Part model, mm, in its own coordinate system. Face numbers are marked on the shaded views. A direction names the side the tool comes from. Round coordinates to 2 decimals unless told otherwise and drop trailing zeros. Write each loop counter-clockwise with the first axis right and the second up, starting at its lowest first coordinate (ties: lowest second). Pieces come first, ordered by that corner, then holes.
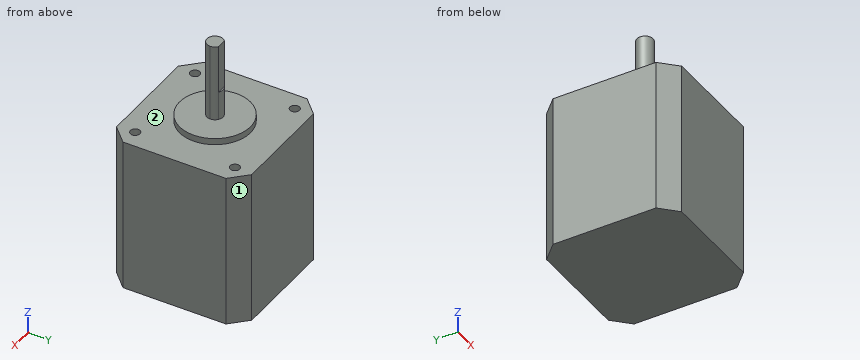
from build123d import *

# Parameters (mm, degrees)
SKETCH1_R           = 11
SKETCH1_R_2         = 1.5
SKETCH1_R_3         = 2.5
BOSS_EXTRUDE1_DEPTH = 48
SKETCH1_3_R         = 11
SKETCH1_3_R_2       = 2.5
BOSS_EXTRUDE2_DEPTH = 2
BOSS_EXTRUDE3_DEPTH = 26
BOSS_EXTRUDE4_DEPTH = 11
SKETCH1_6_R         = 1.5
CUT_EXTRUDE1_DEPTH  = 5


with BuildPart() as part:
    # Sketch1 → Boss-Extrude1 (new body)
    # profile 1 of 10: a face of its own
    with BuildSketch(Plane.XY):
        Polygon((-16, -21), (-21, -16), (-21, 16), (-16, 21), (16, 21), (21, 16), (21, -16), (16, -21), align=None)
        Circle(SKETCH1_R, mode=Mode.SUBTRACT)
        with Locations((15.5, -15.5)):
            Circle(SKETCH1_R_2, mode=Mode.SUBTRACT)
        with Locations((-15.5, -15.5)):
            Circle(SKETCH1_R_2, mode=Mode.SUBTRACT)
        with Locations((15.5, 15.5)):
            Circle(SKETCH1_R_2, mode=Mode.SUBTRACT)
        with Locations((-15.5, 15.5)):
            Circle(SKETCH1_R_2, mode=Mode.SUBTRACT)
    # profile 2 of 10: a face of its own
    with BuildSketch(Plane.XY):
        Circle(SKETCH1_R)
        Circle(SKETCH1_R_3, mode=Mode.SUBTRACT)
    # profile 3 of 10: a face of its own
    with BuildSketch(Plane.XY):
        with BuildLine():
            ThreePointArc((1.5, 2), (0, 2.5), (-1.5, 2))
            Line((-1.5, 2), (1.5, 2))
        make_face()
    # profile 4 of 10: a face of its own
    with BuildSketch(Plane.XY):
        with BuildLine():
            Line((1.5, 2), (-1.5, 2))
            ThreePointArc((-1.5, 2), (-1.118033989, -2.236067977), (2.5, 0))
            ThreePointArc((2.5, 0), (2.236067977, 1.118033989), (1.5, 2))
        make_face()
    # profile 5 of 10: a face of its own
    with BuildSketch(Plane.XY):
        with BuildLine():
            ThreePointArc((1.5, 2), (0, 2.5), (-1.5, 2))
            Line((-1.5, 2), (1.5, 2))
        make_face()
    # profile 6 of 10: a face of its own
    with BuildSketch(Plane.XY):
        with BuildLine():
            Line((1.5, 2), (-1.5, 2))
            ThreePointArc((-1.5, 2), (-1.118033989, -2.236067977), (2.5, 0))
            ThreePointArc((2.5, 0), (2.236067977, 1.118033989), (1.5, 2))
        make_face()
    # profile 7 of 10: a face of its own
    with BuildSketch(Plane.XY):
        with Locations((-15.5, -15.5)):
            Circle(SKETCH1_R_2)
    # profile 8 of 10: a face of its own
    with BuildSketch(Plane.XY):
        with Locations((15.5, -15.5)):
            Circle(SKETCH1_R_2)
    # profile 9 of 10: a face of its own
    with BuildSketch(Plane.XY):
        with Locations((15.5, 15.5)):
            Circle(SKETCH1_R_2)
    # profile 10 of 10: a face of its own
    with BuildSketch(Plane.XY):
        with Locations((-15.5, 15.5)):
            Circle(SKETCH1_R_2)
    extrude(amount=-BOSS_EXTRUDE1_DEPTH)

    # Sketch1_3 → Boss-Extrude2 (add)
    with BuildSketch(Plane.XY):
        Circle(SKETCH1_3_R)
        Circle(SKETCH1_3_R_2, mode=Mode.SUBTRACT)
    extrude(amount=BOSS_EXTRUDE2_DEPTH)

    # Sketch1_4 → Boss-Extrude3 (add)
    with BuildSketch(Plane.XY):
        with BuildLine():
            Line((1.5, 2), (-1.5, 2))
            ThreePointArc((-1.5, 2), (-1.118033989, -2.236067977), (2.5, 0))
            ThreePointArc((2.5, 0), (2.236067977, 1.118033989), (1.5, 2))
        make_face()
    extrude(amount=BOSS_EXTRUDE3_DEPTH)

    # Sketch1_5 → Boss-Extrude4 (add)
    with BuildSketch(Plane.XY):
        with BuildLine():
            ThreePointArc((1.5, 2), (0, 2.5), (-1.5, 2))
            Line((-1.5, 2), (1.5, 2))
        make_face()
        with BuildLine():
            Line((1.5, 2), (-1.5, 2))
            ThreePointArc((-1.5, 2), (-1.118033989, -2.236067977), (2.5, 0))
            ThreePointArc((2.5, 0), (2.236067977, 1.118033989), (1.5, 2))
        make_face()
    extrude(amount=BOSS_EXTRUDE4_DEPTH)

    # Sketch1_6 → Cut-Extrude1 (cut)
    with BuildSketch(Plane.XY):
        with Locations((-15.5, 15.5)):
            Circle(SKETCH1_6_R)
        with Locations((15.5, 15.5)):
            Circle(SKETCH1_6_R)
        with Locations((15.5, -15.5)):
            Circle(SKETCH1_6_R)
        with Locations((-15.5, -15.5)):
            Circle(SKETCH1_6_R)
    extrude(amount=-CUT_EXTRUDE1_DEPTH, mode=Mode.SUBTRACT)


solid = part.part
Q1. Tool access for the marked faces 1 and 2: list every direction of +Z, -Z, +X, -X, +Y, -Y with a clear straight run to the whole face (end or side of a thin tool).
Q2. Wall check: line 1 (Y direction, x = -15.5, z = -1.45); line 2 (Y direction, x = 15, z = -2); line 3 (Z direction, x = -14.5, y = -4). Give the ranges that are in metal, low to high.
Q3. Saw through at A-A, the plane x = 0. Write the cut outline in (y, z), and give its area (3 significant figures).
Q4. Drop flat-ended pins along their axis: P1, Ø2.5, axis at x = 16, y = 15.5, coming from the +Z side; P2, Ø17.5, axis at x = -2, y = -4, coming from the +Z side; P3, Ø2.5, axis at x = -15.5, y = -15.5, coming from the +Z side; P4, Ø12, axis at x = -0.5, y = 16, coming from the +Z side. Give the stop position or say it passes through.
Q5. Saw through at C-C, the plane y = -9. Write the cut outline in (x, z), and give its area (3 significant figures).
Q6. Saw through at D-D, the plane y = -18. Write the cut outline in (x, z), and give its area (3 significant figures).
Q7. Saw through at B-B, the plane z = -21. Write the cut outline in (x, y), and give its area (3 significant figures).
Computed:
1. face 1: +Z, -Z, +X, +Y
1. face 2: +Z
2. line 1: y = -21 to -17, -14 to 14, 17 to 21
2. line 2: y = -21 to -16.91, -14.09 to 14.09, 16.91 to 21
2. line 3: z = -48 to 0
3. outline: (-21, -48) - (21, -48) - (21, 0) - (11, 0) - (11, 2) - (2.5, 2) - (2.5, 11) - (2, 11) - (2, 26) - (-2.5, 26) - (-2.5, 2) - (-11, 2) - (-11, 0) - (-21, 0) - close
3. area: 2,170 mm2
4. P1: stops at z = 0
4. P2: stops at z = 26
4. P3: stops at z = -5
4. P4: stops at z = 2
5. outline: (-21, -48) - (21, -48) - (21, 0) - (6.32, 0) - (6.32, 2) - (-6.32, 2) - (-6.32, 0) - (-21, 0) - close
5. area: 2,040 mm2
6. outline: (-19, -48) - (19, -48) - (19, 0) - (-19, 0) - close
6. area: 1,820 mm2
7. outline: (-21, -16) - (-16, -21) - (16, -21) - (21, -16) - (21, 16) - (16, 21) - (-16, 21) - (-21, 16) - close
7. area: 1,710 mm2
